```python
from build123d import *

# Parameters (mm, degrees)
BOSS_EXTRUDE3_DEPTH       = 7.9375
SKETCH5_R                 = 3.4925
CUT_EXTRUDE4_DEPTH        = 33.489674755
SKETCH6_R                 = 14.3002
CUT_EXTRUDE5_DEPTH        = 2.159
TAP_DRILL_FOR_3_48_TAP2_D = 1.9939
F_10_CLEARANCE_HOLE1_D    = 5.1054
FILLET1_R                 = 2.032
FILLET2_R                 = 0.508


with BuildPart() as part:
    # Sketch1 → Boss-Extrude3 (new body)
    with BuildSketch(Plane(origin=(0, 0, 0), x_dir=(0, 0, -1), z_dir=(1, 0, 0))):
        with BuildLine():
            Line((9.216458059, 14.457106413), (23.495, 5.354483857))
            ThreePointArc((23.495, 5.354483857), (26.431497015, 0), (23.495, -5.354483857))
            Line((23.495, -5.354483857), (9.216458059, -14.457106413))
            ThreePointArc((9.216458059, -14.457106413), (0, -17.145), (-9.216458059, -14.457106413))
            Line((-9.216458059, -14.457106413), (-23.495, -5.354483857))
            ThreePointArc((-23.495, -5.354483857), (-26.431497015, 0), (-23.495, 5.354483857))
            Line((-23.495, 5.354483857), (-9.216458059, 14.457106413))
            ThreePointArc((-9.216458059, 14.457106413), (0, 17.145), (9.216458059, 14.457106413))
        make_face()
    extrude(amount=BOSS_EXTRUDE3_DEPTH)

    # Sketch5 → Cut-Extrude4 (cut, through all)
    with BuildSketch(Plane(origin=(7.9375, 0, 0), x_dir=(0, 0, -1), z_dir=(1, 0, 0))):
        Circle(SKETCH5_R)
    extrude(amount=-CUT_EXTRUDE4_DEPTH, mode=Mode.SUBTRACT)

    # Sketch6 → Cut-Extrude5 (cut)
    with BuildSketch(Plane(origin=(7.9375, 0, 0), x_dir=(0, 0, -1), z_dir=(1, 0, 0))):
        Circle(SKETCH6_R)
    extrude(amount=-CUT_EXTRUDE5_DEPTH, mode=Mode.SUBTRACT)

    # Tap Drill for #3-48 Tap2 (through all)
    with Locations(Plane(origin=(5.7785, 0, 0), x_dir=(0, 0, -1), z_dir=(1, 0, 0))):
        with Locations((-1.292324468, 7.329136259), (1.292324468, -7.329136259)):
            Hole(TAP_DRILL_FOR_3_48_TAP2_D / 2)

    # #10 Clearance Hole1 (through all)
    with Locations(Plane(origin=(7.9375, 0, 0), x_dir=(0, 0, -1), z_dir=(1, 0, 0))):
        with Locations((-20.955, 0), (20.955, 0), (9.900488765, 18.695562828)):
            Hole(F_10_CLEARANCE_HOLE1_D / 2)

    # Fillet1
    fillet1_edges = [part.edges().sort_by_distance(p)[0] for p in [
        (0, 9.905795135, 16.355729029),
        (0, 17.145, 0),
        (0, 9.905795135, -16.355729029),
        (0, 0, -26.431497015),
        (0, -9.905795135, -16.355729029),
        (0, -17.145, 0),
        (0, -9.905795135, 16.355729029),
        (0, 0, 26.431497015),
    ]]
    fillet(fillet1_edges, radius=FILLET1_R)

    # Fillet2
    fillet2_edges = [part.edges().sort_by_distance(p)[0] for p in [
        (7.9375, 0, 26.431497015),
        (7.9375, -9.905795135, 16.355729029),
        (7.9375, -17.145, 0),
        (7.9375, -9.905795135, -16.355729029),
        (7.9375, 0, -26.431497015),
        (7.9375, 9.905795135, -16.355729029),
        (7.9375, 0, 14.3002),
        (7.9375, 17.145, 0),
        (7.9375, 9.905795135, 16.355729029),
    ]]
    fillet(fillet2_edges, radius=FILLET2_R)


solid = part.part
```
Build history of the part. All positions in model axes, mm. A direction names the side the tool comes from. Round coordinates to 2 decimals unless told otherwise and drop trailing zeros. Order: outer loops, then holes, each group sorted by start corner. A loop starts at its lowest first (then second) coordinate and runs counter-clockwise, first axis right, second up. Notation, with made-up numbers: (60.5, 15.5) -> (82.5, 15.5) arc R16 cw to (82.5, 20.5) -> close; hole circle Ø11 at (38.25, -6). An arc over 180 degrees is marked (long way). Answer in a Markdown table with one row per item.
1) Band-saw the part on B-B on x = 5.25. Give the number of separate pieces and of enclosed holes in the cut face, and give its area (3 significant figures).
Values:
| item | result |
|---|---|
| separate pieces | 1 |
| enclosed holes | 5 |
| area | 1,120 mm2 |
2) Wall check: L1, parallel to Y at x = 5, z = 2; L2, parallel to X at y = -7, z = -8.5; L3, parallel to Z at x = 3.5, y = 7.5. Give the ranges that are in metal, low to high.
Values:
| item | result |
|---|---|
| L1 | -17.03 to -2.86, 2.86 to 6.63, 8.03 to 17.03 |
| L2 | 0 to 5.78 |
| L3 | -20.13 to 0.31, 2.27 to 20.13 |
3) Which spindle directions (+Z, -Z, +X, -X, +Y, -Y) get a long thin tool onto all of the face, cutting with end or side? Do faces 4 (the flat face through (7.938, -15, 2)), 5 (the cylindrical face through (6.62, -13.96, 3.1)). Say none if no direction does.
Values:
| item | result |
|---|---|
| face 4 | +Z, -Z, +X, +Y, -Y |
| face 5 | +X |
4) Band-saw the part on A-A on y = 0. Give the cut face in (x, z).
Values:
| item | result |
|---|---|
| outline | (0, -24.4) arc R2.03 ccw to (2.03, -26.43) -> (7.43, -26.43) arc R0.51 ccw to (7.94, -25.92) -> (7.94, -23.51) -> (0, -23.51) -> close; (0, -18.4) -> (7.94, -18.4) -> (7.94, -14.81) arc R0.51 ccw to (7.43, -14.3) -> (5.78, -14.3) -> (5.78, -3.49) -> (0, -3.49) -> close; (0, 3.49) -> (5.78, 3.49) -> (5.78, 14.3) -> (7.43, 14.3) arc R0.51 ccw to (7.94, 14.81) -> (7.94, 18.4) -> (0, 18.4) -> close; (0, 23.51) -> (7.94, 23.51) -> (7.94, 25.92) arc R0.51 ccw to (7.43, 26.43) -> (2.03, 26.43) arc R2.03 ccw to (0, 24.4) -> close |
5) Pin check, flat tips, straight feed: P1, Ø1, axis at y = -7, z = -10.5, coming from the +X side; P2, Ø1, axis at x = 2, z = 10, coming from the -Y side; P3, Ø3, axis at x = 5.5, y = -4.5, coming from the +Z side. Stop position of each tip, or through.
Values:
| item | result |
|---|---|
| P1 | x = 5.78 |
| P2 | y = -14.28 |
| P3 | z = 25.68 |
6) Mould opens along Z. For faces 1 (the cylindrical face through (0.58, -9.45, -15.93)), 2 (the cylindrical face through (3.913, 0.112, 18.405)), 3 (the cylindrical face through (0.58, 9.45, 15.93)) say: released by +Z, released by -Z, zero draft, split by the parting line, or undercut.
Values:
| item | result |
|---|---|
| face 1 | released by -Z |
| face 2 | undercut |
| face 3 | released by +Z |
